from build123d import *

# Parameters (mm, degrees)
SKETCH_1_W               = 120
SKETCH_1_H               = 120
EXTRUDE_1_DEPTH          = 5
SKETCH_2_W               = 60
SKETCH_2_H               = 60
SKETCH_2_W_2             = 54
SKETCH_2_H_2             = 54
EXTRUDE_2_DEPTH          = 2000
FILLET_1_R               = 5
SKETCH_3_R               = 5
CUT_EXTRUDE_1_DEPTH      = 2000
EXTRUDE_5_DEPTH          = 7.5
PATTERN_LINEAR_1_COUNT   = 2
PATTERN_LINEAR_1_PITCH   = 1500
SKETCH_7_R               = 12.5
EXTRUDE_6_DEPTH          = 30
SKETCH_8_R               = 4
EXTRUDE_7_DEPTH          = 35
PATTERN_LINEAR_2_COUNT   = 2
PATTERN_LINEAR_2_PITCH   = 1500
MIRROR_1_COPY_1_DEPTH    = 7.5
MIRROR_1_COPY_2_SKETCH_R = 12.5
MIRROR_1_COPY_2_DEPTH    = 30
MIRROR_1_COPY_3_SKETCH_R = 4
MIRROR_1_COPY_3_DEPTH    = 35


with BuildPart() as part:
    # 草图1 → 凸台-拉伸1 (new body)
    with BuildSketch(Plane(origin=(0, 0, 0), x_dir=(1, 0, 0), z_dir=(0, 1, 0))):
        Rectangle(SKETCH_1_W, SKETCH_1_H)
    extrude(amount=EXTRUDE_1_DEPTH)

    # 草图2 → 凸台-拉伸2 (add)
    with BuildSketch(Plane(origin=(0, 5, 0), x_dir=(1, 0, 0), z_dir=(0, 1, 0))):
        Rectangle(SKETCH_2_W, SKETCH_2_H)
        Rectangle(SKETCH_2_W_2, SKETCH_2_H_2, mode=Mode.SUBTRACT)
    extrude(amount=EXTRUDE_2_DEPTH)

    # 圆角1
    fillet_1_edges = [part.edges().sort_by_distance(p)[0] for p in [
        (30, 1005, -30),
        (-30, 1005, -30),
        (-30, 1005, 30),
        (30, 1005, 30),
    ]]
    fillet(fillet_1_edges, radius=FILLET_1_R)

    # 草图3 → 切除-拉伸1 (cut)
    with BuildSketch(Plane(origin=(0, 5, 0), x_dir=(1, 0, 0), z_dir=(0, 1, 0))):
        with Locations(Location((-45, 45, 0), (0, 0, 270))):
            Circle(SKETCH_3_R)
        with Locations(Location((45, 45, 0), (0, 0, 270))):
            Circle(SKETCH_3_R)
        with Locations(Location((-45, -45, 0), (0, 0, 270))):
            Circle(SKETCH_3_R)
        with Locations(Location((45, -45, 0), (0, 0, 270))):
            Circle(SKETCH_3_R)
    extrude(amount=-CUT_EXTRUDE_1_DEPTH, mode=Mode.SUBTRACT)

    # 草图6 → 凸台-拉伸5 (add, symmetric)
    with BuildSketch(Plane(origin=(0, 0, 0), x_dir=(0, 0, -1), z_dir=(1, 0, 0))):
        Polygon((30, 1785), (30, 1725), (40, 1725), (40, 1755), (33, 1755), (33, 1785), align=None)
    extrude_5 = extrude(amount=EXTRUDE_5_DEPTH, both=True)

    # 阵列(线性)1: 凸台-拉伸5 ×2
    with Locations(*[(0, -i * PATTERN_LINEAR_1_PITCH, 0) for i in range(1, PATTERN_LINEAR_1_COUNT)]):
        add(extrude_5)

    # 草图7 → 凸台-拉伸6 (add)
    with BuildSketch(Plane(origin=(0, 1755, 0), x_dir=(1, 0, 0), z_dir=(0, 1, 0))):
        with Locations((0, 52)):
            Circle(SKETCH_7_R)
    extrude_6 = extrude(amount=-EXTRUDE_6_DEPTH)

    # 草图8 → 凸台-拉伸7 (add)
    with BuildSketch(Plane(origin=(0, 1755, 0), x_dir=(1, 0, 0), z_dir=(0, 1, 0))):
        with Locations(Location((0, 50, 0), (0, 0, 90))):
            Circle(SKETCH_8_R)
    extrude_7 = extrude(amount=EXTRUDE_7_DEPTH)

    # 阵列(线性)2: 凸台-拉伸6, 凸台-拉伸7 ×2
    with Locations(*[(0, -i * PATTERN_LINEAR_2_PITCH, 0) for i in range(1, PATTERN_LINEAR_2_COUNT)]):
        add(extrude_6)
        add(extrude_7)

    # 镜向1: 凸台-拉伸5, 凸台-拉伸6, 凸台-拉伸7 across plane
    add(extrude_5.mirror(Plane(origin=(0, 0, 0), x_dir=(1, 0, 0), z_dir=(0, 0, -1))))
    add(extrude_6.mirror(Plane(origin=(0, 0, 0), x_dir=(1, 0, 0), z_dir=(0, 0, -1))))
    add(extrude_7.mirror(Plane(origin=(0, 0, 0), x_dir=(1, 0, 0), z_dir=(0, 0, -1))))

    # 镜向1 copy 1 sketch → 镜向1 copy 1 (add, symmetric)
    with BuildSketch(Plane(origin=(0, -1500, 0), x_dir=(0, 0, 1), z_dir=(1, 0, 0))):
        Polygon((30, -1785), (30, -1725), (40, -1725), (40, -1755), (33, -1755), (33, -1785), align=None)
    extrude(amount=MIRROR_1_COPY_1_DEPTH, both=True)

    # 镜向1 copy 2 sketch → 镜向1 copy 2 (add)
    with BuildSketch(Plane(origin=(0, 255, 0), x_dir=(1, 0, 0), z_dir=(0, 1, 0))):
        with Locations((0, -52)):
            Circle(MIRROR_1_COPY_2_SKETCH_R)
    extrude(amount=-MIRROR_1_COPY_2_DEPTH)

    # 镜向1 copy 3 sketch → 镜向1 copy 3 (add)
    with BuildSketch(Plane(origin=(0, 255, 0), x_dir=(1, 0, 0), z_dir=(0, 1, 0))):
        with Locations((0, -50)):
            Circle(MIRROR_1_COPY_3_SKETCH_R)
    extrude(amount=MIRROR_1_COPY_3_DEPTH)


solid = part.part
Can you work these out from the model? Positions are in its coordinate system, mm. A direction names the side the tool comes from. Coordinates: 2 decimals unless noted, no trailing zeros. Loops run counter-clockwise (first coordinate to the right, second up) from the corner with the lowest first, then second, coordinate; pieces in that order, holes last. Notation, with made-up numbers: (19.5, 53.5) - (76.5, 53.5) arc R30 ccw to (76.5, 82.5) - close; hole circle Ø3 at (-35.5, 84.25). An arc over 180 degrees is marked (long way). Answer as a JSON object with one key per item and string values. Group by question number.
Item 1: If I drill on L1, parallel to X at y = 1, z = 45; L2, parallel to X at y = 903.5, z = -11.5; L3, parallel to Y at x = 3.5, z = 30.5, over which ranges is the centre line in solid material (lowest first)? Write a range as from..to.
Item 2: If we mould it in two halves opening along Y, with no side actions, what happens to faces 1 (the face through (0, 2005, -29)), 2 (the face through (-1, 0, -1)), 3 (the face through (0, 991, -30))? For each: released by +Y, released by -Y, zero draft, split by the parting line, or undercut.
Item 3: For pin 1 (12 mm diameter, centred on x = -20, y = 504, fed in from -Z); pin 2 (4 mm diameter, centred on x = -1.5, z = -10, fed in from +Y); pin 3 (5 mm diameter, centred on y = 585, z = -8.5, fed in from +X), each with a flat end and sliding along its axis, tell me the tip position at first contact or that it passes through.
Item 4: If we section it at A-A (y = 626.5): List the corners of the cut face in (x, z) for me.
Item 5: On a 3-axis mill with a long thin cutter (end or side, diameter ignored), from which of +Z, -Z, +X, -X, +Y, -Y can I reach the whole of each face in a straight line? I mean faces 4 (the face through (30, 991, 0)), 5 (the face through (-30, 991, 0)), 6 (the face through (0, 991, -27)). Say none if no direction works.
Returned:
{
 "1": {"L1": "x = -60..-50, -40..40, 50..60", "L2": "x = -30..-27, 27..30", "L3": "y = 0..5, 225..285, 1725..1785"},
 "2": {"face 1": "released by +Y", "face 2": "released by -Y", "face 3": "undercut"},
 "3": {"pin 1": "stops at z = -30", "pin 2": "stops at y = 5", "pin 3": "stops at x = 30"},
 "4": {"outline": "(-30, -25) arc R5 ccw to (-25, -30) - (25, -30) arc R5 ccw to (30, -25) - (30, 25) arc R5 ccw to (25, 30) - (-25, 30) arc R5 ccw to (-30, 25) - close; hole (-27, -27) - (27, -27) - (27, 27) - (-27, 27) - close"},
 "5": {"face 4": "+Z, -Z, +X, +Y", "face 5": "+Z, -Z, -X, +Y", "face 6": "+Y"}
}
